Check sheet for the modelled part. Datum: model origin and axes. Units: mm. A direction names the side the tool comes from. Round coordinates to 2 decimals unless told otherwise and drop trailing zeros. Order: outer loops, then holes, each group sorted by start corner. A loop starts at its lowest first (then second) coordinate and runs counter-clockwise, first axis right, second up.
Q1. Cross-section at B-B on x = -19. Record the cut outline in (y, z).
Q2. Cross-section at D-D on z = 37.5. Record the cut outline in (x, y), then the cut area to 3 significant figures.
Q3. Mould release check, pull along Z, two halves, no side actions. Record for faces 1 (the flat face through (19, 0, 12)), 2 (the flat face through (-13, 0, 35)), 3 (the cylindrical face through (-0.38, 0.21, 79.71)), 4 (the cylindrical face through (18.62, 0.21, 79.71)): +Z half, -Z half, draft (parallel to the pull), parting line (faces both ways), or undercut.
Q4. Cross-section at C-C on y = 2. Record the cut outline in (x, z), then the cut area to 3 significant figures.
Q5. Depth check by flat-ended pin: P1, Ø3, axis at x = -1, y = 1.5, coming from the -Z side; P2, Ø6.5, axis at x = 20, y = 0, coming from the -Z side. Enter the tip coordinate at first touch or a pass-through.
Q6. Set-up check for faces 5 (the flat face through (25, 0, 41)), 6 (the flat face through (-19, 0, 12)), 7 (the flat face through (0, 0, 72)): record each of +Z, -Z, +X, -X, +Y, -Y from which the full face is reachable in a straight line by a thin tool's end or side.
Q7. Scan lines: probe 1 along Z at (x, y) = (19, 7); probe 2 along X at (y, z) = (4.25, 78); probe 3 along X at (y, z) = (-5.75, 20). Record each from-to range of solid material in increasing order.
Q8. Cross-section at A-A on z = 20. Record the cut outline in (x, y).
from build123d import *

# Parameters (mm, degrees)
SKETCH_1_W          = 50
SKETCH_1_H          = 30
EXTRUDE_1_DEPTH     = 84
SKETCH_2_W          = 26
SKETCH_2_H          = 14
CUT_EXTRUDE_1_DEPTH = 72
SKETCH_5_W          = 12
SKETCH_5_H          = 8
CUT_EXTRUDE_4_DEPTH = 13
SKETCH_6_W          = 12
SKETCH_6_H          = 8
CUT_EXTRUDE_5_DEPTH = 13
SKETCH_7_R          = 1.75
CUT_EXTRUDE_7_DEPTH = 31


with BuildPart() as part:
    # ｽｹｯﾁ1 → ﾎﾞｽ - 押し出し1 (new body)
    with BuildSketch(Plane.XY):
        Rectangle(SKETCH_1_W, SKETCH_1_H)
    extrude(amount=EXTRUDE_1_DEPTH)

    # ｽｹｯﾁ2 → ｶｯﾄ - 押し出し1 (cut)
    with BuildSketch(Plane(origin=(0, 0, 0), x_dir=(-1, 0, 0), z_dir=(0, 0, -1))):
        Rectangle(SKETCH_2_W, SKETCH_2_H)
    extrude(amount=-CUT_EXTRUDE_1_DEPTH, mode=Mode.SUBTRACT)

    # ｽｹｯﾁ5 → ｶｯﾄ - 押し出し4 (cut, through all)
    with BuildSketch(Plane.ZY.offset(-13)):
        with Locations((6, 0)):
            Rectangle(SKETCH_5_W, SKETCH_5_H)
    extrude(amount=-CUT_EXTRUDE_4_DEPTH, mode=Mode.SUBTRACT)

    # ｽｹｯﾁ6 → ｶｯﾄ - 押し出し5 (cut, through all)
    with BuildSketch(Plane(origin=(-13, 0, 0), x_dir=(0, 0, -1), z_dir=(1, 0, 0))):
        with Locations((-6, 0)):
            Rectangle(SKETCH_6_W, SKETCH_6_H)
    extrude(amount=-CUT_EXTRUDE_5_DEPTH, mode=Mode.SUBTRACT)

    # ｽｹｯﾁ7 → ｶｯﾄ - 押し出し7 (cut, through all)
    with BuildSketch(Plane(origin=(0, 15, 0), x_dir=(1, 0, 0), z_dir=(0, 1, 0))):
        with Locations((19, -20)):
            Circle(SKETCH_7_R)
        with Locations((19, -43)):
            Circle(SKETCH_7_R)
        with Locations((19, -78)):
            Circle(SKETCH_7_R)
        with Locations((0, -78)):
            Circle(SKETCH_7_R)
        with Locations((-19, -78)):
            Circle(SKETCH_7_R)
        with Locations((-19, -43)):
            Circle(SKETCH_7_R)
        with Locations((-19, -20)):
            Circle(SKETCH_7_R)
    extrude(amount=-CUT_EXTRUDE_7_DEPTH, mode=Mode.SUBTRACT)


solid = part.part
Results found:
1. outline: (-15, 0) - (-4, 0) - (-4, 12) - (4, 12) - (4, 0) - (15, 0) - (15, 18.25) - (-15, 18.25) - close; (-15, 21.75) - (15, 21.75) - (15, 41.25) - (-15, 41.25) - close; (-15, 44.75) - (15, 44.75) - (15, 76.25) - (-15, 76.25) - close; (-15, 79.75) - (15, 79.75) - (15, 84) - (-15, 84) - close
2. outline: (-25, -15) - (25, -15) - (25, 15) - (-25, 15) - close; hole (-13, -7) - (13, -7) - (13, 7) - (-13, 7) - close
2. area: 1,140 mm2
3. face 1: -Z half
3. face 2: draft
3. face 3: undercut
3. face 4: undercut
4. outline: (-25, 12) - (-13, 12) - (-13, 72) - (13, 72) - (13, 12) - (25, 12) - (25, 84) - (-25, 84) - close; hole circle Ø3.5 at (-19, 20); hole circle Ø3.5 at (-19, 43); hole circle Ø3.5 at (-19, 78); hole circle Ø3.5 at (0, 78); hole circle Ø3.5 at (19, 20); hole circle Ø3.5 at (19, 43); hole circle Ø3.5 at (19, 78)
4. area: 1,970 mm2
5. P1: stops at z = 72
5. P2: stops at z = 12
6. face 5: +Z, -Z, +X, +Y, -Y
6. face 6: -Z, +X, -X
6. face 7: -Z
7. probe 1: z = 0 to 18.25, 21.75 to 41.25, 44.75 to 76.25, 79.75 to 84
7. probe 2: x = -25 to -20.75, -17.25 to -1.75, 1.75 to 17.25, 20.75 to 25
7. probe 3: x = -25 to -20.75, -17.25 to -13, 13 to 17.25, 20.75 to 25
8. outline: (-25, -15) - (-20.75, -15) - (-20.75, 15) - (-25, 15) - close; (-17.25, -15) - (17.25, -15) - (17.25, 15) - (-17.25, 15) - close; (20.75, -15) - (25, -15) - (25, 15) - (20.75, 15) - close; hole (-13, -7) - (13, -7) - (13, 7) - (-13, 7) - close
